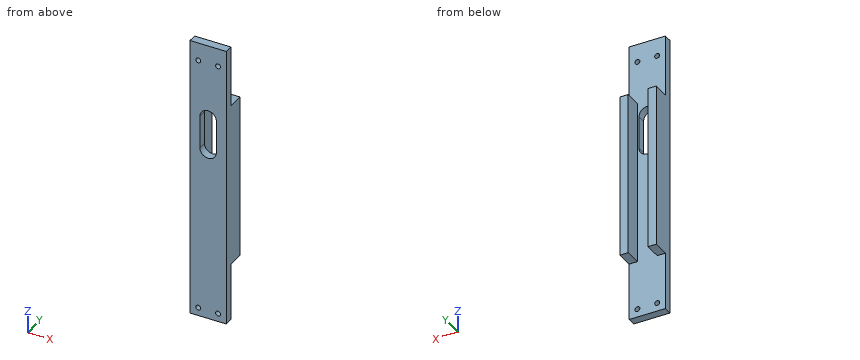
```python
from build123d import *

# Parameters (mm, degrees)
SKETCH1_W           = 22
SKETCH1_H           = 166.3
SKETCH1_R           = 1.5
BOSS_EXTRUDE1_DEPTH = 5
CUT_EXTRUDE1_DEPTH  = 5
SKETCH3_W           = 22
SKETCH3_H           = 5
BOSS_EXTRUDE2_DEPTH = 6
SKETCH4_W           = 5
SKETCH4_H           = 100
BOSS_EXTRUDE3_DEPTH = 10


with BuildPart() as part:
    # Sketch1 → Boss-Extrude1 (new body)
    with BuildSketch(Plane(origin=(0, 0, 0), x_dir=(1, 0, 0), z_dir=(0, 1, 0))):
        with Locations((11, 83.15)):
            Rectangle(SKETCH1_W, SKETCH1_H)
        with Locations(Location((5, 161.3, 0), (0, 0, 270))):
            Circle(SKETCH1_R, mode=Mode.SUBTRACT)
        with Locations(Location((17, 161.3, 0), (0, 0, 270))):
            Circle(SKETCH1_R, mode=Mode.SUBTRACT)
        with Locations(Location((17, 5, 0), (0, 0, 270))):
            Circle(SKETCH1_R, mode=Mode.SUBTRACT)
        with Locations(Location((5, 5, 0), (0, 0, 270))):
            Circle(SKETCH1_R, mode=Mode.SUBTRACT)
    extrude(amount=BOSS_EXTRUDE1_DEPTH)

    # Sketch2 → Cut-Extrude1 (cut)
    with BuildSketch(Plane(origin=(0, 0, 0), x_dir=(-1, 0, 0), z_dir=(0, -1, 0))):
        with BuildLine():
            Line((-16, 40), (-16, 60))
            ThreePointArc((-16, 60), (-11, 65), (-6, 60))
            Line((-6, 60), (-6, 40))
            ThreePointArc((-6, 40), (-11, 35), (-16, 40))
        make_face()
    extrude(amount=-CUT_EXTRUDE1_DEPTH, mode=Mode.SUBTRACT)

    # Sketch3 → Boss-Extrude2 (add)
    with BuildSketch(Plane.XY):
        with Locations((11, 2.5)):
            Rectangle(SKETCH3_W, SKETCH3_H)
    extrude(amount=BOSS_EXTRUDE2_DEPTH)

    # Sketch4 → Boss-Extrude3 (add)
    with BuildSketch(Plane(origin=(0, 5, 0), x_dir=(1, 0, 0), z_dir=(0, 1, 0))):
        with Locations((2.5, 81.3)):
            Rectangle(SKETCH4_W, SKETCH4_H)
        with Locations((19.5, 81.3)):
            Rectangle(SKETCH4_W, SKETCH4_H)
    extrude(amount=BOSS_EXTRUDE3_DEPTH)


solid = part.part
```
Source: CAD feature listing. Evaluate the final solid. Frame: model axes, mm. Coordinates: 2 decimals unless noted, no trailing zeros. Loops run counter-clockwise (first coordinate to the right, second up) from the corner with the lowest first, then second, coordinate; pieces in that order, holes last. Notation, with made-up numbers: M -10,57.5 L 24,57.5 A6 cw 24,61.5 Z; hole C 66.25,-28.75 d10. An arc over 180 degrees is marked long. Put each result on its own line as item: value. Start each with the question number.
1) Cut plane A-A on z = -5. Return the cut outline in (x, y).
2) Ray query, L1, parallel to X at y = 3.4, z = -161.3; L2, parallel to X at y = 2.25, z = -52.5; L3, parallel to Z at x = 18.25, y = 13.25. Return the intervals inside material, ascending. Write a range as from..to.
3) Contact query for flat-ended pins moving along their axis: pin 1 Ø1 at (y, z) = (8.5, -121.5) entering from -X; pin 2 Ø3.5 at (x, z) = (17, -5) entering from +Y; pin 3 Ø4 at (x, y) = (20, 11) entering from +Z; pin 4 Ø4 at (x, y) = (19, 11.5) entering from -Z. Output: stop coordinate, or through.
4) Cut plane C-C on x = 11. Return the cut outline in (y, z).
5) Cut plane B-B on y = 13.25. Return the cut outline in (x, z).
6) Cut plane D-D on y = 1.75. Return the cut outline in (x, z).
The answers:
1. outline: M 0,0 L 3.5,0 L 3.5,5 L 0,5 Z; M 6.5,0 L 15.5,0 L 15.5,5 L 6.5,5 Z; M 18.5,0 L 22,0 L 22,5 L 18.5,5 Z
2. L1: x = 0..3.5, 6.5..15.5, 18.5..22
2. L2: x = 0..6, 16..22
2. L3: z = -131.3..-31.3
3. pin 1: stops at x = 0
3. pin 2: stops at y = 5
3. pin 3: stops at z = -31.3
3. pin 4: stops at z = -131.3
4. outline: M 0,-166.3 L 5,-166.3 L 5,-65 L 0,-65 Z; M 0,-35 L 5,-35 L 5,6 L 0,6 Z
5. outline: M 0,-131.3 L 5,-131.3 L 5,-31.3 L 0,-31.3 Z; M 17,-131.3 L 22,-131.3 L 22,-31.3 L 17,-31.3 Z
6. outline: M 0,-166.3 L 22,-166.3 L 22,6 L 0,6 Z; hole C 5,-161.3 d3; hole C 5,-5 d3; hole M 6,-60 A5 ccw 16,-60 L 16,-40 A5 ccw 6,-40 Z; hole C 17,-161.3 d3; hole C 17,-5 d3
